Verification items for the finished model (mm, model axes). A direction names the side the tool comes from. Coordinates: 2 decimals unless noted, no trailing zeros. Write each loop counter-clockwise with the first axis right and the second up, starting at its lowest first coordinate (ties: lowest second). Pieces come first, ordered by that corner, then holes. Notation, with made-up numbers: (-5.5, 82) -> (44.5, 82) arc R33 ccw to (44.5, 116) -> close; hole circle Ø8 at (-14, -15). An arc over 180 degrees is marked (long way). Write item = value, one per line. Start each with the question number.
(1) Gauge pin test, flat ends, axial feed: pin 1 Ø6 at (x, y) = (-60, 7.5) entering from +Z; pin 2 Ø2 at (x, y) = (-29, -17) entering from +Z; pin 3 Ø10 at (y, z) = (-41.5, -44) entering from +X; pin 4 Ø6 at (x, z) = (54, -28) entering from -Y. Record the tip position at first contact, or that the pin passes through.
(2) Section check C-C (z = -28). Record the cut outline in (x, y), plus the area to 3 significant figures.
(3) Section check A-A (x = -54). Record the cut outline in (y, z), plus the area to 3 significant figures.
(4) Material ranges on probe 1 along X at (y, z) = (11.75, -28); probe 2 along Z at (x, y) = (54, 6); probe 3 along X at (y, z) = (-4, -37), recorded low to high. Write a range as [from, to].
(5) Section check D-D (y = 3.5). Record the cut outline in (x, z).
(6) Mould release check, pull along X, two halves, no side actions. Record for faces 5 (the face through (70, 15, -28)), 6 (the face through (27.6, -22.21, -24)), 7 (the face through (-35, -20, -38)), 8 (the face through (20, -20, -38)): released by +X, released by -X, zero draft, split by the parting line, or undercut.
(7) Section check B-B (y = -21). Record the cut outline in (x, z), plus the area to 3 significant figures.
(8) Set-up check for faces 1 (the face through (60, 15, 0)), 2 (the face through (-60, 15, 0)), 3 (the face through (35, -20, -38)), 4 (the face through (38.508, 15.21, 5.068)): record each of +Z, -Z, +X, -X, +Y, -Y from which the full face is reachable in a straight line by a thin tool's end or side.
```python
from build123d import *

# Parameters (mm, degrees)
F0_R     = 5
F3_DEPTH = 30
F4_R     = 15
F2_R     = 5
F5_DEPTH = 15


with BuildPart() as f3:
    # F0 (on Front) → F3 (new body)
    with BuildSketch(Plane.XZ):
        with BuildLine():
            ThreePointArc((28.7228132327, 0), (0, 55), (-28.7228132327, 0))
            Line((-28.7228132327, 0), (0, 0))
            Line((0, 0), (28.7228132327, 0))
        make_face()
        with BuildLine():
            ThreePointArc((20, 20), (14.1421356237, 5.8578643763), (0, 0))
            ThreePointArc((0, 0), (-14.1421356237, 34.1421356237), (20, 20))
        make_face(mode=Mode.SUBTRACT)
        Polygon((-28.7228132327, 0), (-70, 0), (-70, -56), (70, -56), (70, 0), (28.7228132327, 0), (0, 0), align=None)
        with Locations((-54, -28)):
            Circle(F0_R, mode=Mode.SUBTRACT)
        with Locations((54, -28)):
            Circle(F0_R, mode=Mode.SUBTRACT)
    extrude(amount=-F3_DEPTH)

    # F4
    f4_edges = [f3.edges().sort_by_distance(p)[0] for p in [
        (-28.722813, 15, 0),
        (28.722813, 15, 0),
    ]]
    fillet(f4_edges, radius=F4_R)

    # F2 (on plane+point) → F5 (join)
    with BuildSketch(Plane.YZ.offset(-35)):
        with BuildLine():
            Line((0, -56), (0, -11))
            Line((0, -11), (-45.0515173064, -37.369694507))
            ThreePointArc((-45.0515173064, -37.369694507), (-49.6515038966, -48.6169586422), (-40, -56))
            Line((-40, -56), (0, -56))
        make_face()
        with Locations((-40, -46)):
            Circle(F2_R, mode=Mode.SUBTRACT)
    extrude(amount=F5_DEPTH)

    # F6: F3 across plane


with BuildPart() as f3_1:
    add(f3.part)
    add(f3.part.mirror(Plane.YZ))


solid = f3_1.part
```
Response:
q1.pin_1 = 0
q1.pin_2 = -20.37
q1.pin_3 = 35
q1.pin_4 = through
q2.outline = (-70, 0) -> (-59, 0) -> (-59, 30) -> (-70, 30) -> close; (-49, 0) -> (-35, 0) -> (-35, -29.04) -> (-20, -29.04) -> (-20, 0) -> (20, 0) -> (20, -29.04) -> (35, -29.04) -> (35, 0) -> (49, 0) -> (49, 30) -> (-49, 30) -> close; (59, 0) -> (70, 0) -> (70, 30) -> (59, 30) -> close
q2.area = 4,470 mm2
q3.outline = (0, -56) -> (30, -56) -> (30, -33) -> (0, -33) -> close; (0, -23) -> (30, -23) -> (30, 0) -> (0, 0) -> close
q3.area = 1,380 mm2
q4.probe_1 = [-70, -59], [-49, 49], [59, 70]
q4.probe_2 = [-56, -33], [-23, 0]
q4.probe_3 = [-35, -20], [20, 35]
q5.outline = (-70, -56) -> (70, -56) -> (70, 0) -> (49.75, 0) arc R15 cw to (34.82, 16.5) arc R35 ccw (long way) to (-34.82, 16.5) arc R15 cw to (-49.75, 0) -> (-70, 0) -> close; hole circle Ø10 at (-54, -28); hole circle Ø40 at (0, 20); hole circle Ø10 at (54, -28)
q6.face_5 = released by +X
q6.face_6 = zero draft
q6.face_7 = released by -X
q6.face_8 = undercut
q7.outline = (-35, -56) -> (-20, -56) -> (-20, -23.29) -> (-35, -23.29) -> close; (20, -56) -> (35, -56) -> (35, -23.29) -> (20, -23.29) -> close
q7.area = 981 mm2
q8.face_1 = +Z, +X, +Y, -Y
q8.face_2 = +Z, -X, +Y, -Y
q8.face_3 = +Z, -Z, +X, -Y
q8.face_4 = +X, +Y, -Y
